from build123d import *

# Parameters (mm, degrees)
F1_DEPTH      = 76.2
F2_W          = 28.575
F2_H          = 57.15
F3_DEPTH      = 38.063829867
F3_DEPTH_BACK = 25.4
F4_R          = 4.699
F5_DEPTH      = 19.051


with BuildPart() as f1:
    # F0 (on Right) → F1 (new body)
    with BuildSketch(Plane.YZ):
        Polygon((-57.187170133, 0), (-57.187170133, -19.05), (38.062829867, -19.05), (38.062829867, 0), (12.662829867, 0), (12.662829867, 50.8), (-12.737170133, 50.8), (-12.737170133, 0), align=None)
    extrude(amount=F1_DEPTH)

    # F2 (on Front) → F3 (cut, two sides)
    with BuildSketch(Plane.XZ) as f3_sk:
        with Locations((38.1, 50.8)):
            Rectangle(F2_W, F2_H)
    extrude(amount=-F3_DEPTH, mode=Mode.SUBTRACT)
    extrude(f3_sk.sketch, amount=F3_DEPTH_BACK, mode=Mode.SUBTRACT)

    # F4 (on Top) → F5 (cut, through all)
    with BuildSketch(Plane.XY):
        with Locations((12.7, 25.362829867)):
            Circle(F4_R)
        with Locations((63.5, 25.362829867)):
            Circle(F4_R)
        with Locations((12.7, -44.487170133)):
            Circle(F4_R)
        with Locations((63.5, -44.487170133)):
            Circle(F4_R)
    extrude(amount=-F5_DEPTH, mode=Mode.SUBTRACT)


solid = f1.part
For this review, take the finished solid that the model builds, in its own axes (mm). A direction names the side the tool comes from. Round coordinates to 2 decimals unless told otherwise and drop trailing zeros. Order: outer loops, then holes, each group sorted by start corner. A loop starts at its lowest first (then second) coordinate and runs counter-clockwise, first axis right, second up. Notation, with made-up numbers: M 57.5,84 L 64.5,84 A4 ccw 64.5,90 Z; hole C 3,-8 d11. An arc over 180 degrees is marked long. Use a Markdown table: item, result. Add a question column.
Item 1: Add section A-A, the plane z = 42.5. Give the boundary of the cut face in (x, y), then the cut area to 3 significant figures.
Item 2: Mouldability with a two-part tool opening along X and no side actions: class faces 1 (the flat face through (0, 0, 9)), 2 (the flat face through (38, 12.663, 19)), 3 (the cylindrical face through (11.681, -49.074, -9.392)) as released by +X, released by -X, zero draft, split by the parting line, or undercut.
Item 3: Tool access review of faces 4 (the flat face through (38, 26, 0)), 5 (the flat face through (64, 0, 50.8)), 6 (the flat face through (38, -35, 0)), 7 (the flat face through (38, 0, 22.225)): name each direction out of +Z, -Z, +X, -X, +Y, -Y from which nothing blocks a thin tool from reaching the whole face with its end or side.
Item 4: Add section B-B, the plane x = 63.5. Give the boundary of the cut face in (y, z), then the cut area to 3 significant figures.
Item 5: Add section D-D, the plane x = 32.5. Give the boundary of the cut face in (y, z) (3 decimals), then the cut area to 3 significant figures.
Item 6: To check wall thickness, follow line 1 along Y through (x, z) = (12.7, -12.75); line 2 along Y through (x, z) = (12, -13); line 3 along Z through (x, y) = (44, 4) (3 decimals). State the ranges of each line that lie inside material, in increasing order.
Item 7: Add section C-C, the plane y = 28.5. Give the boundary of the cut face in (x, z).
Item 8: Insertion check: pin 1 (1 mm diameter, centred on x = 46, y = -8, fed in from +Z) (3 decimals); pin 2 (8 mm diameter, centred on x = 29, z = 16.5, fed in from +Y); pin 3 (4 mm diameter, centred on x = 28.5, y = -26.5, fed in from +Z). Each pin has a flat end and moves straight along its axis. Give the tip position at first contact, or say it passes through.
Geometry results:
| question | item | result |
|---|---|---|
| 1 | outline | M 0,-12.74 L 23.81,-12.74 L 23.81,12.66 L 0,12.66 Z; M 52.39,-12.74 L 76.2,-12.74 L 76.2,12.66 L 52.39,12.66 Z |
| 1 | area | 1,210 mm² |
| 2 | face 1 | released by -X |
| 2 | face 2 | zero draft |
| 2 | face 3 | undercut |
| 3 | face 4 | +Z, +X, -X, +Y |
| 3 | face 5 | +Z, +X, -X, +Y, -Y |
| 3 | face 6 | +Z, +X, -X, -Y |
| 3 | face 7 | +Z, +Y, -Y |
| 4 | outline | M -57.19,-19.05 L -49.19,-19.05 L -49.19,0 L -57.19,0 Z; M -39.79,-19.05 L 20.66,-19.05 L 20.66,0 L 12.66,0 L 12.66,50.8 L -12.74,50.8 L -12.74,0 L -39.79,0 Z; M 30.06,-19.05 L 38.06,-19.05 L 38.06,0 L 30.06,0 Z |
| 4 | area | 2,750 mm² |
| 5 | outline | M -57.187,-19.05 L 38.063,-19.05 L 38.063,0 L 12.663,0 L 12.663,22.225 L -12.737,22.225 L -12.737,0 L -57.187,0 Z |
| 5 | area | 2,380 mm² |
| 6 | line 1 | y = -57.19 to -49.19, -39.79 to 20.66, 30.06 to 38.06 |
| 6 | line 2 | y = -57.19 to -49.13, -39.84 to 20.72, 30.01 to 38.06 |
| 6 | line 3 | z = -19.05 to 22.225 |
| 7 | outline | M 0,-19.05 L 9.2,-19.05 L 9.2,0 L 0,0 Z; M 16.2,-19.05 L 60,-19.05 L 60,0 L 16.2,0 Z; M 67,-19.05 L 76.2,-19.05 L 76.2,0 L 67,0 Z |
| 8 | pin 1 | stops at z = 22.225 |
| 8 | pin 2 | stops at y = 12.66 |
| 8 | pin 3 | stops at z = 0 |
